```python
from build123d import *

# Parameters (mm, degrees)
BOSS_EXTRUDE1_DEPTH = 33
SKETCH3_W           = 4.5
SKETCH3_H           = 4.99999
SKETCH3_W_2         = 3
SKETCH3_H_2         = 0.5
SKETCH4_R           = 1.25
CUT_EXTRUDE1_DEPTH  = 45.395945761
SKETCH5_R           = 3.25
SKETCH5_R_2         = 4.75
CUT_EXTRUDE2_DEPTH  = 3.5
SKETCH6_W           = 8
SKETCH6_H           = 8
CUT_EXTRUDE3_DEPTH  = 3.5
SKETCH7_W           = 6.5
SKETCH7_H           = 1.5
SKETCH7_W_2         = 2.5
SKETCH7_H_2         = 25
SKETCH8_R           = 2.742
SKETCH8_R_2         = 1.25
BOSS_EXTRUDE2_DEPTH = 2.992
SKETCH8_3_R         = 1.25
BOSS_EXTRUDE3_DEPTH = 21.336
CUT_EXTRUDE4_DEPTH  = 1.016


with BuildPart() as part:
    # Sketch1 → Boss-Extrude1 (new body)
    with BuildSketch(Plane(origin=(0, 0, 0), x_dir=(1, 0, 0), z_dir=(0, 1, 0))):
        Polygon((-18, 21), (-21, 18), (-21, -18), (-18, -21), (18, -21), (21, -18), (21, 18), (18, 21), align=None)
    extrude(amount=BOSS_EXTRUDE1_DEPTH)

    # Sketch3 → Cut-Revolve2 (revolve, cut)
    with BuildSketch(Plane(origin=(0, 0, 0), x_dir=(0.7071067811865481, 0, -0.7071067811865469), z_dir=(0.7071067811865469, 0, 0.7071067811865481)), mode=Mode.PRIVATE) as cut_revolve2_sk:
        with Locations((2.25, 30.500005)):
            Rectangle(SKETCH3_W, SKETCH3_H)
        Polygon((29.355164466, 12.5), (27.577164466, 12.5), (25.577164466, 12.5), (25.577164466, 21), (27.577164466, 21), (29.355164466, 21), align=None)
        with Locations((12.5, 32.75)):
            Rectangle(SKETCH3_W_2, SKETCH3_H_2)
    revolve(cut_revolve2_sk.sketch.rotate(Axis((0, 33, 0), (0, -1, 0)), 225), axis=Axis((0, 33, 0), (0, -1, 0)), mode=Mode.SUBTRACT)

    # Sketch4 → Cut-Extrude1 (cut, through all)
    with BuildSketch(Plane(origin=(0, 33, 0), x_dir=(1, 0, 0), z_dir=(0, 1, 0))):
        with Locations(Location((-15.5, 15.5, 0), (0, 0, 270))):
            Circle(SKETCH4_R)
        with Locations(Location((15.5, 15.5, 0), (0, 0, 270))):
            Circle(SKETCH4_R)
        with Locations(Location((15.5, -15.5, 0), (0, 0, 270))):
            Circle(SKETCH4_R)
        with Locations(Location((-15.5, -15.5, 0), (0, 0, 270))):
            Circle(SKETCH4_R)
    extrude(amount=-CUT_EXTRUDE1_DEPTH, mode=Mode.SUBTRACT)

    # Sketch5 → Cut-Extrude2 (cut)
    with BuildSketch(Plane.XZ):
        with Locations(Location((-15.5, 15.5, 0), (0, 0, 270))):
            Circle(SKETCH5_R)
        with Locations(Location((-15.5, -15.5, 0), (0, 0, 270))):
            Circle(SKETCH5_R)
        with Locations(Location((15.5, -15.5, 0), (0, 0, 270))):
            Circle(SKETCH5_R)
        with Locations(Location((15.5, 15.5, 0), (0, 0, 270))):
            Circle(SKETCH5_R)
        with Locations(Location((0, 0, 0), (0, 0, 270))):
            Circle(SKETCH5_R_2)
    extrude(amount=-CUT_EXTRUDE2_DEPTH, mode=Mode.SUBTRACT)

    # Sketch6 → Cut-Extrude3 (cut)
    with BuildSketch(Plane(origin=(21, 0, 0), x_dir=(0, 0, -1), z_dir=(1, 0, 0))):
        with Locations((0, 6.5)):
            Rectangle(SKETCH6_W, SKETCH6_H)
    extrude(amount=-CUT_EXTRUDE3_DEPTH, mode=Mode.SUBTRACT)

    # Sketch7 → Revolve1 (revolve)
    with BuildSketch(Plane(origin=(0, 0, 0), x_dir=(0.7071067811865481, 0, -0.7071067811865469), z_dir=(0.7071067811865469, 0, 0.7071067811865481)), mode=Mode.PRIVATE) as revolve1_sk:
        with Locations((7.75, 33.75)):
            Rectangle(SKETCH7_W, SKETCH7_H)
        with Locations((1.25, 40.50001)):
            Rectangle(SKETCH7_W_2, SKETCH7_H_2)
    revolve(revolve1_sk.sketch.rotate(Axis((0, 33, 0), (0, -1, 0)), 225), axis=Axis((0, 33, 0), (0, -1, 0)))



with BuildPart() as body_2:
    # Sketch8 → Boss-Extrude2 (new body)
    with BuildSketch(Plane.XZ):
        with Locations(Location((-15.5, 15.5, 0), (0, 0, 270))):
            Circle(SKETCH8_R)
        with Locations(Location((-15.5, 15.5, 0), (0, 0, 90))):
            Circle(SKETCH8_R_2, mode=Mode.SUBTRACT)
        with Locations(Location((-15.5, 15.5, 0), (0, 0, 90))):
            Circle(SKETCH8_R_2)
        with Locations(Location((15.5, 15.5, 0), (0, 0, 270))):
            Circle(SKETCH8_R)
        with Locations(Location((15.5, 15.5, 0), (0, 0, 90))):
            Circle(SKETCH8_R_2, mode=Mode.SUBTRACT)
        with Locations(Location((15.5, 15.5, 0), (0, 0, 90))):
            Circle(SKETCH8_R_2)
        with Locations(Location((15.5, -15.5, 0), (0, 0, 270))):
            Circle(SKETCH8_R)
        with Locations(Location((15.5, -15.5, 0), (0, 0, 90))):
            Circle(SKETCH8_R_2, mode=Mode.SUBTRACT)
        with Locations(Location((15.5, -15.5, 0), (0, 0, 90))):
            Circle(SKETCH8_R_2)
        with Locations(Location((-15.5, -15.5, 0), (0, 0, 270))):
            Circle(SKETCH8_R)
        with Locations(Location((-15.5, -15.5, 0), (0, 0, 90))):
            Circle(SKETCH8_R_2, mode=Mode.SUBTRACT)
        with Locations(Location((-15.5, -15.5, 0), (0, 0, 90))):
            Circle(SKETCH8_R_2)
    extrude(amount=-BOSS_EXTRUDE2_DEPTH)


with BuildPart() as part_1:
    add(part.part)

    add(body_2.part)  # Boss-Extrude3 merges body 2
    # Sketch8<3> → Boss-Extrude3 (add)
    with BuildSketch(Plane.XZ):
        with Locations(Location((-15.5, 15.5, 0), (0, 0, 270))):
            Circle(SKETCH8_3_R)
        with Locations(Location((-15.5, -15.5, 0), (0, 0, 270))):
            Circle(SKETCH8_3_R)
        with Locations(Location((15.5, -15.5, 0), (0, 0, 270))):
            Circle(SKETCH8_3_R)
        with Locations(Location((15.5, 15.5, 0), (0, 0, 270))):
            Circle(SKETCH8_3_R)
    extrude(amount=-BOSS_EXTRUDE3_DEPTH)

    # Sketch9 → Cut-Extrude4 (cut)
    with BuildSketch(Plane.XZ):
        with BuildLine():
            Line((16.262, -16.262), (18.133993166, -16.262))
            ThreePointArc((18.133993166, -16.262), (18.214864017, -15.884808224), (18.242, -15.5))
            ThreePointArc((18.242, -15.5), (18.214864017, -15.115191776), (18.133993166, -14.738))
            Line((18.133993166, -14.738), (16.262, -14.738))
            Line((16.262, -14.738), (16.262, -12.866006834))
            ThreePointArc((16.262, -12.866006834), (15.5, -12.758), (14.738, -12.866006834))
            Line((14.738, -12.866006834), (14.738, -14.738))
            Line((14.738, -14.738), (12.866006834, -14.738))
            ThreePointArc((12.866006834, -14.738), (12.758, -15.5), (12.866006834, -16.262))
            Line((12.866006834, -16.262), (14.738, -16.262))
            Line((14.738, -16.262), (14.738, -18.133993166))
            ThreePointArc((14.738, -18.133993166), (15.5, -18.242), (16.262, -18.133993166))
            Line((16.262, -18.133993166), (16.262, -16.262))
        make_face()
        with BuildLine():
            ThreePointArc((-12.758, -15.5), (-12.785135983, -15.115191776), (-12.866006834, -14.738))
            Line((-12.866006834, -14.738), (-14.738, -14.738))
            Line((-14.738, -14.738), (-14.738, -12.866006834))
            ThreePointArc((-14.738, -12.866006834), (-15.5, -12.758), (-16.262, -12.866006834))
            Line((-16.262, -12.866006834), (-16.262, -14.738))
            Line((-16.262, -14.738), (-18.133993166, -14.738))
            ThreePointArc((-18.133993166, -14.738), (-18.242, -15.5), (-18.133993166, -16.262))
            Line((-18.133993166, -16.262), (-16.262, -16.262))
            Line((-16.262, -16.262), (-16.262, -18.133993166))
            ThreePointArc((-16.262, -18.133993166), (-15.5, -18.242), (-14.738, -18.133993166))
            Line((-14.738, -18.133993166), (-14.738, -16.262))
            Line((-14.738, -16.262), (-12.866006834, -16.262))
            ThreePointArc((-12.866006834, -16.262), (-12.785135983, -15.884808224), (-12.758, -15.5))
        make_face()
        with BuildLine():
            Line((-16.262, 16.262), (-18.133993166, 16.262))
            ThreePointArc((-18.133993166, 16.262), (-18.242, 15.5), (-18.133993166, 14.738))
            Line((-18.133993166, 14.738), (-16.262, 14.738))
            Line((-16.262, 14.738), (-16.262, 12.866006834))
            ThreePointArc((-16.262, 12.866006834), (-15.5, 12.758), (-14.738, 12.866006834))
            Line((-14.738, 12.866006834), (-14.738, 14.738))
            Line((-14.738, 14.738), (-12.866006834, 14.738))
            ThreePointArc((-12.866006834, 14.738), (-12.785135983, 15.115191776), (-12.758, 15.5))
            ThreePointArc((-12.758, 15.5), (-12.785135983, 15.884808224), (-12.866006834, 16.262))
            Line((-12.866006834, 16.262), (-14.738, 16.262))
            Line((-14.738, 16.262), (-14.738, 18.133993166))
            ThreePointArc((-14.738, 18.133993166), (-15.5, 18.242), (-16.262, 18.133993166))
            Line((-16.262, 18.133993166), (-16.262, 16.262))
        make_face()
        with BuildLine():
            ThreePointArc((12.866006834, 16.262), (12.758, 15.5), (12.866006834, 14.738))
            Line((12.866006834, 14.738), (14.738, 14.738))
            Line((14.738, 14.738), (14.738, 12.866006834))
            ThreePointArc((14.738, 12.866006834), (15.5, 12.758), (16.262, 12.866006834))
            Line((16.262, 12.866006834), (16.262, 14.738))
            Line((16.262, 14.738), (18.133993166, 14.738))
            ThreePointArc((18.133993166, 14.738), (18.214864017, 15.115191776), (18.242, 15.5))
            ThreePointArc((18.242, 15.5), (18.214864017, 15.884808224), (18.133993166, 16.262))
            Line((18.133993166, 16.262), (16.262, 16.262))
            Line((16.262, 16.262), (16.262, 18.133993166))
            ThreePointArc((16.262, 18.133993166), (15.5, 18.242), (14.738, 18.133993166))
            Line((14.738, 18.133993166), (14.738, 16.262))
            Line((14.738, 16.262), (12.866006834, 16.262))
        make_face()
    extrude(amount=-CUT_EXTRUDE4_DEPTH, mode=Mode.SUBTRACT)


solid = part_1.part
```
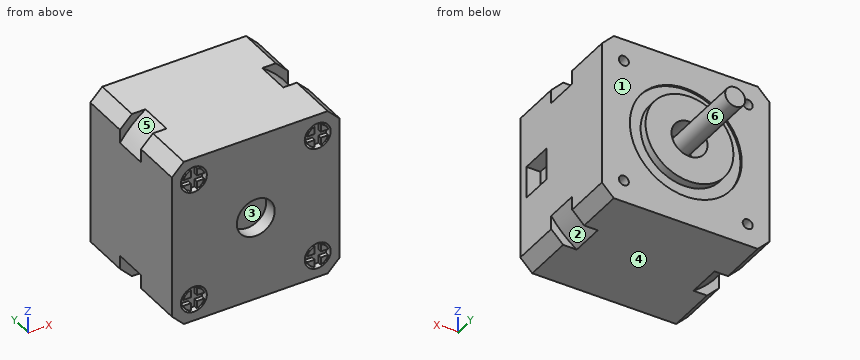
The listing builds one solid part. Answer for the finished solid, in the listing's coordinates (mm). Face numbers are marked on the shaded views. A direction names the side the tool comes from. Coordinates: 2 decimals unless noted, no trailing zeros. Loops run counter-clockwise (first coordinate to the right, second up) from the corner with the lowest first, then second, coordinate; pieces in that order, holes last. Notation, with made-up numbers: (43.25, 15) -> (72.25, 15) arc R26 ccw to (72.25, 39) -> close; hole circle Ø6 at (43, 74.25). An arc over 180 degrees is marked (long way). Use one line per item in the form item = value. Start each with the question number.
Item 1: The mould has two halves that part along X. Classify the marked faces 1, 2 and 3: released by +X, released by -X, zero draft, split by the parting line, or undercut.
Item 2: Flat-ended cylindrical pins translate along their axes: pin 1 Ø12 at (x, z) = (-12.5, -3.5) entering from +Y; pin 2 Ø1.9 at (x, z) = (-17, -18) entering from +Y; pin 3 Ø2 at (x, z) = (15.5, -15.5) entering from +Y. Find the tip coordinate at first contact, or state that the pin passes through.
Item 3: Consider L1, parallel to X at y = 26.5, z = -15.5; L2, parallel to X at y = 32.9, z = 0; L3, parallel to X at y = 2.15, z = 15.5. Determine where each line is inside the solid, lowest interval first. Write a range as [from, to].
Item 4: The part is cut by section A-A on x = 0. Determine the outline of the cut face in (y, z), then the cut area to 3 significant figures.
Item 5: The part is cut by section D-D on z = -9. Determine the outline of the cut face in (x, y), then the cut area to 3 significant figures.
Item 6: A tool of negligible diameter and unlimited length cuts with its end or side. For the marked faces 4, 5 and 6, from which of +Z, -Z, +X, -X, +Y, -Y can it reach the whole face along a straight path? Write none if from no direction.
Item 7: The part is cut by section C-C on z = 0. Determine the outline of the cut face in (x, y), then the cut area to 3 significant figures.
Item 8: The part is cut by section B-B on y = 18. Determine the outline of the cut face in (x, z), then the cut area to 3 significant figures.
Answer key:
q1.face_1 = zero draft
q1.face_2 = released by +X
q1.face_3 = undercut
q2.pin_1 = 34.5
q2.pin_2 = 33
q2.pin_3 = 21.34
q3.L1 = [-21, -16.75], [-14.25, 14.25], [16.75, 21]
q3.L2 = [-21, -14], [-11, -4.5], [-2.5, 2.5], [4.5, 11], [14, 21]
q3.L3 = [-21, -18.75], [-18.24, -12.76], [-12.25, 12.25], [12.76, 18.24], [18.75, 21]
q4.outline = (0, -21) -> (33, -21) -> (33, -14) -> (32.5, -14) -> (32.5, -11) -> (34.5, -11) -> (34.5, -4.5) -> (28, -4.5) -> (28, -2.5) -> (53, -2.5) -> (53, 2.5) -> (28, 2.5) -> (28, 4.5) -> (34.5, 4.5) -> (34.5, 11) -> (32.5, 11) -> (32.5, 14) -> (33, 14) -> (33, 21) -> (0, 21) -> (0, 4.75) -> (3.5, 4.75) -> (3.5, -4.75) -> (0, -4.75) -> close
q4.area = 1,450 mm2
q5.outline = (-21, 0) -> (21, 0) -> (21, 33) -> (10.72, 33) -> (10.72, 32.5) -> (6.32, 32.5) -> (6.32, 34.5) -> (-6.32, 34.5) -> (-6.32, 32.5) -> (-10.72, 32.5) -> (-10.72, 33) -> (-21, 33) -> close
q5.area = 1,400 mm2
q6.face_4 = -Z, +X, -X, +Y, -Y
q6.face_5 = +Z, -X
q6.face_6 = +Y
q7.outline = (-21, 0) -> (-4.75, 0) -> (-4.75, 3.5) -> (4.75, 3.5) -> (4.75, 0) -> (21, 0) -> (21, 2.5) -> (17.5, 2.5) -> (17.5, 10.5) -> (21, 10.5) -> (21, 33) -> (14, 33) -> (14, 32.5) -> (11, 32.5) -> (11, 34.5) -> (4.5, 34.5) -> (4.5, 28) -> (2.5, 28) -> (2.5, 53) -> (-2.5, 53) -> (-2.5, 28) -> (-4.5, 28) -> (-4.5, 34.5) -> (-11, 34.5) -> (-11, 32.5) -> (-14, 32.5) -> (-14, 33) -> (-21, 33) -> close
q7.area = 1,420 mm2
q8.outline = (-21, -14.6) arc R25.58 ccw to (-14.6, -21) -> (14.6, -21) arc R25.58 ccw to (21, -14.6) -> (21, 14.6) arc R25.58 ccw to (14.6, 21) -> (-14.6, 21) arc R25.58 ccw to (-21, 14.6) -> close
q8.area = 1,690 mm2
